Work out the finished part from the listing and answer in its coordinate system (mm). A direction names the side the tool comes from. Coordinates: 2 decimals unless noted, no trailing zeros. Order: outer loops, then holes, each group sorted by start corner. A loop starts at its lowest first (then second) coordinate and runs counter-clockwise, first axis right, second up.
1. A tool of negligible diameter and unlimited length cuts with its end or side. For faces 1 (the flat face through (8, 5, -28)), 2 (the flat face through (18, 5, 30.607)), 3 (the cylindrical face through (-29.87, 4.93, -2.79)), 4 (the flat face through (9, 5, -7.607)), from which of +Z, -Z, +X, -X, +Y, -Y can it reach the whole face along a straight path? Write none if from no direction.
2. Flat-ended cylindrical pins translate along their axes: pin 1 Ø3 at (y, z) = (6.5, 28) entering from +X; pin 2 Ø5 at (x, y) = (32, 7) entering from -Z; pin 3 Ø2 at (y, z) = (6.5, 2) entering from +X. Find the tip coordinate at first contact, or state that the pin passes through.
3. The part is cut by section A-A, the plane x = 33. Give the vertices of the cut face in (y, z), then the cut area to 3 significant figures.
4. The part is cut by section D-D, the plane x = 18. Give the vertices of the cut face in (y, z), then the cut area to 3 significant figures.
5. The part is cut by section B-B, the plane z = -17. Give the vertices of the cut face in (x, y), then the cut area to 3 significant figures.
6. The part is cut by section C-C, the plane x = 8.5. Give the vertices of the cut face in (y, z).
7. Find the intervals of material crossed by probe 1 along Z at (x, y) = (-34.5, 1.5); probe 2 along Z at (x, y) = (29.5, 3.25); probe 3 along X at (y, z) = (5.5, -29), in increasing order.
8. Determine the mould class of faces 5 (the flat face through (16, 5, 5)), 6 (the flat face through (0, 0, -1)), 7 (the flat face through (-31.7, 4.9, 18.3)) for opening direction X: +X half, -X half, draft (parallel to the pull), parting line (faces both ways), or undercut.
```python
from build123d import *

# Parameters (mm, degrees)
BOSS_EXTRUDE1_DEPTH = 10


with BuildPart() as part:
    # Sketch1 → Boss-Extrude1 (new body)
    with BuildSketch(Plane(origin=(0, 0, 0), x_dir=(1, 0, 0), z_dir=(0, 1, 0))):
        with BuildLine():
            Line((-10, 43.284271247), (-10, 28.284271247))
            ThreePointArc((-10, 28.284271247), (-12.552949398, 27.247448714), (-15, 25.980762114))
            Line((-15, 25.980762114), (-21.642135624, 37.485278485))
            Line((-21.642135624, 37.485278485), (-30.302389662, 32.485278485))
            Line((-30.302389662, 32.485278485), (-22.802389662, 19.494897428))
            ThreePointArc((-22.802389662, 19.494897428), (-24.494897428, 17.320508076), (-25.980762114, 15))
            Line((-25.980762114, 15), (-37.485278485, 21.642135624))
            Line((-37.485278485, 21.642135624), (-42.485278485, 12.981881586))
            Line((-42.485278485, 12.981881586), (-29.494897428, 5.481881586))
            ThreePointArc((-29.494897428, 5.481881586), (-29.873457473, 2.752551286), (-30, 0))
            Line((-30, 0), (-43.284271247, 0))
            Line((-43.284271247, 0), (-43.284271247, -10))
            Line((-43.284271247, -10), (-28.284271247, -10))
            ThreePointArc((-28.284271247, -10), (-27.247448714, -12.552949398), (-25.980762114, -15))
            Line((-25.980762114, -15), (-37.485278485, -21.642135624))
            Line((-37.485278485, -21.642135624), (-32.485278485, -30.302389662))
            Line((-32.485278485, -30.302389662), (-19.494897428, -22.802389662))
            ThreePointArc((-19.494897428, -22.802389662), (-17.320508076, -24.494897428), (-15, -25.980762114))
            Line((-15, -25.980762114), (-21.642135624, -37.485278485))
            Line((-21.642135624, -37.485278485), (-12.981881586, -42.485278485))
            Line((-12.981881586, -42.485278485), (-5.481881586, -29.494897428))
            ThreePointArc((-5.481881586, -29.494897428), (-2.752551286, -29.873457473), (0, -30))
            Line((0, -30), (0, -25.980762114))
            Line((0, -25.980762114), (5.980762114, -25.980762114))
            Line((5.980762114, -25.980762114), (10.606601718, -30.606601718))
            Line((10.606601718, -30.606601718), (25.606601718, -30.606601718))
            ThreePointArc((25.606601718, -30.606601718), (40.914600616, -27.351889426), (25.606601718, -24.097177134))
            Line((25.606601718, -24.097177134), (10.606601718, -24.097177134))
            Line((10.606601718, -24.097177134), (0.964787573, -12.606510487))
            Line((0.964787573, -12.606510487), (0.959757824, -9.468981171))
            Line((0.959757824, -9.468981171), (29.777364974, -9.468981171))
            ThreePointArc((29.777364974, -9.468981171), (45.458969743, -7.234490585), (29.777364974, -5))
            Line((29.777364974, -5), (0.952593634, -5))
            Line((0.952593634, -5), (0.940399696, 2.606510487))
            Line((0.940399696, 2.606510487), (15.940399696, 2.606510487))
            ThreePointArc((15.940399696, 2.606510487), (31.551740371, 5.030424476), (15.964787573, 7.606510487))
            Line((15.964787573, 7.606510487), (0.964787573, 7.606510487))
            Line((0.964787573, 7.606510487), (0.964787573, 12.606510487))
            Line((0.964787573, 12.606510487), (10.606601718, 24.097177134))
            Line((10.606601718, 24.097177134), (25.606601718, 24.097177134))
            ThreePointArc((25.606601718, 24.097177134), (40.914600616, 27.351889426), (25.606601718, 30.606601718))
            Line((25.606601718, 30.606601718), (10.606601718, 30.606601718))
            Line((10.606601718, 30.606601718), (5, 25))
            Line((5, 25), (0, 25))
            Line((0, 25), (0, 30))
            Line((0, 30), (0, 43.284271247))
            Line((0, 43.284271247), (-10, 43.284271247))
        make_face()
    extrude(amount=BOSS_EXTRUDE1_DEPTH)


solid = part.part
```
Geometry says:
1. face 1: -Z, +Y, -Y
1. face 2: +Z, +Y, -Y
1. face 3: -X, +Y, -Y
1. face 4: +Y, -Y
2. pin 1: stops at x = 40.91
2. pin 2: stops at z = -35.35
2. pin 3: stops at x = 44.25
3. outline: (0, -35.35) - (10, -35.35) - (10, -19.35) - (0, -19.35) - close; (0, 0.59) - (10, 0.59) - (10, 13.88) - (0, 13.88) - close; (0, 19.35) - (10, 19.35) - (10, 35.35) - (0, 35.35) - close
3. area: 453 mm2
4. outline: (0, -30.61) - (10, -30.61) - (10, -24.1) - (0, -24.1) - close; (0, -10.83) - (10, -10.83) - (10, 0.69) - (0, 0.69) - close; (0, 5) - (10, 5) - (10, 9.47) - (0, 9.47) - close; (0, 24.1) - (10, 24.1) - (10, 30.61) - (0, 30.61) - close
4. area: 290 mm2
5. outline: (-40.17, 0) - (-29.44, 0) - (-29.44, 10) - (-40.17, 10) - close; (-24.72, 0) - (4.65, 0) - (4.65, 10) - (-24.72, 10) - close
5. area: 401 mm2
6. outline: (0, -28.5) - (10, -28.5) - (10, -21.59) - (0, -21.59) - close; (0, -7.61) - (10, -7.61) - (10, -2.61) - (0, -2.61) - close; (0, 5) - (10, 5) - (10, 9.47) - (0, 9.47) - close; (0, 21.59) - (10, 21.59) - (10, 28.5) - (0, 28.5) - close
7. probe 1: z = -19.92 to -8.37, 0 to 10, 19.92 to 26.81
7. probe 2: z = -34.59 to -20.12, -10.42 to 0.28, 5 to 9.47, 20.12 to 34.59
7. probe 3: x = -28.29 to -16.74, -10 to 0, 9 to 40.74
8. face 5: undercut
8. face 6: draft
8. face 7: -X half
